Input: dimensioned drawing with shaded views. Units: mm. Origin: part minimum x, y, z. Give positions to 0.01 mm unless a question says otherwise; leave off trailing zeros. Loops run counter-clockwise (first coordinate to the right, second up) from the corner with the lowest first, then second, coordinate; pieces in that order, holes last. Notation, with made-up numbers: M 45,75 L 62,75 A17 ccw 62,86 Z; hole C -11.5,55.25 d4. An arc over 180 degrees is marked long. Answer in a Markdown table with one row per item.
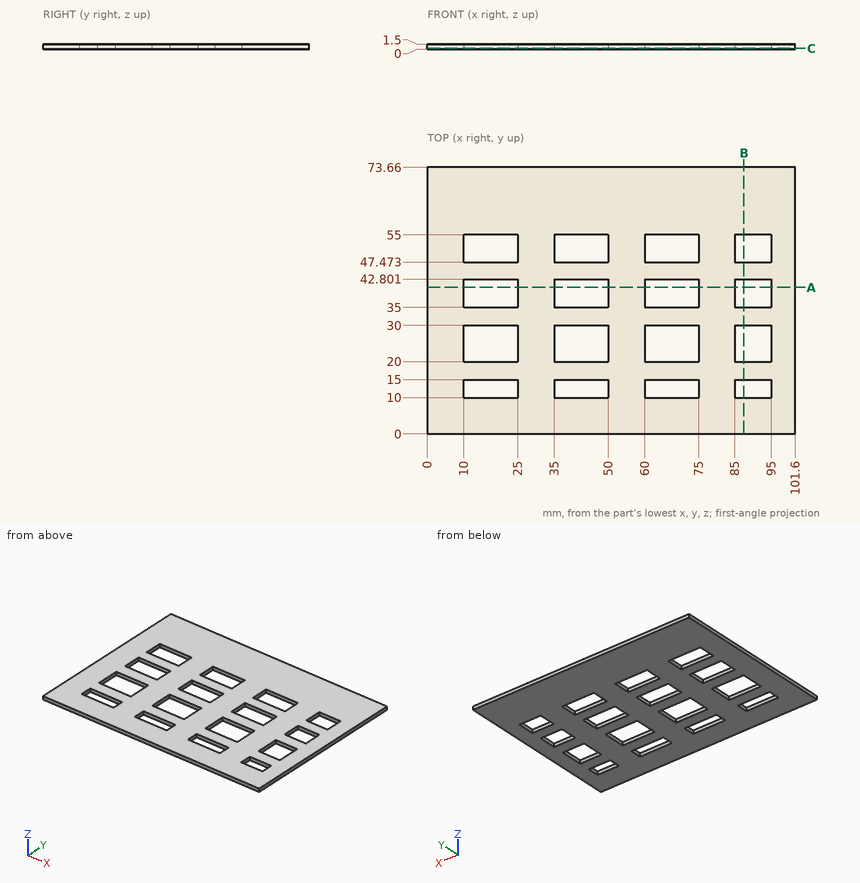
Q1. Section query B-B (x = 87.5). Output: boundary loops of the cut face in (y, z), plus the area to 3 significant figures.
Values follow:
| item | result |
|---|---|
| outline | M 0,0 L 10,0 L 10,1.5 L 0,1.5 Z; M 15,0 L 20,0 L 20,1.5 L 15,1.5 Z; M 30,0 L 35,0 L 35,1.5 L 30,1.5 Z; M 42.8,0 L 47.47,0 L 47.47,1.5 L 42.8,1.5 Z; M 55,0 L 73.66,0 L 73.66,1.5 L 55,1.5 Z |
| area | 65.0 mm^2 |
Q2. Section query C-C (z = 0.3). Give the number of separate pieces and of enclosed holes in the cut face, plus the area to 3 significant figures.
Values follow:
| item | result |
|---|---|
| separate pieces | 1 |
| enclosed holes | 16 |
| area | 5,820 mm^2 |
Q3. Ray query, probe 1 along Y at (x, z) = (23, 0.6); probe 2 along X at (y, z) = (40.5, 0.55). Return the intervals inside material, ascending. Write a range as from..to.
Values follow:
| item | result |
|---|---|
| probe 1 | 0..10, 15..20, 30..35, 42.8..47.47, 55..73.66 |
| probe 2 | 0..10, 25..35, 50..60, 75..85, 95..101.6 |
Q4. Section query A-A (y = 40.5). Output: boundary loops of the cut face in (x, z).
Values follow:
| item | result |
|---|---|
| outline | M 0,0 L 10,0 L 10,1.5 L 0,1.5 Z; M 25,0 L 35,0 L 35,1.5 L 25,1.5 Z; M 50,0 L 60,0 L 60,1.5 L 50,1.5 Z; M 75,0 L 85,0 L 85,1.5 L 75,1.5 Z; M 95,0 L 101.6,0 L 101.6,1.5 L 95,1.5 Z |
